Check sheet for the modelled part. Datum: model origin and axes. Units: mm. Face numbers are marked on the shaded views. Round coordinates to 2 decimals unless told otherwise and drop trailing zeros. Order: outer loops, then holes, each group sorted by start corner. A loop starts at its lowest first (then second) coordinate and runs counter-clockwise, first axis right, second up. Notation, with made-up numbers: (87, 51) -> (99, 51) arc R11 ccw to (99, 61) -> close; hole circle Ø3 at (28, 18.5). An arc over 180 degrees is marked (long way). Answer in a Markdown table with one row per item.
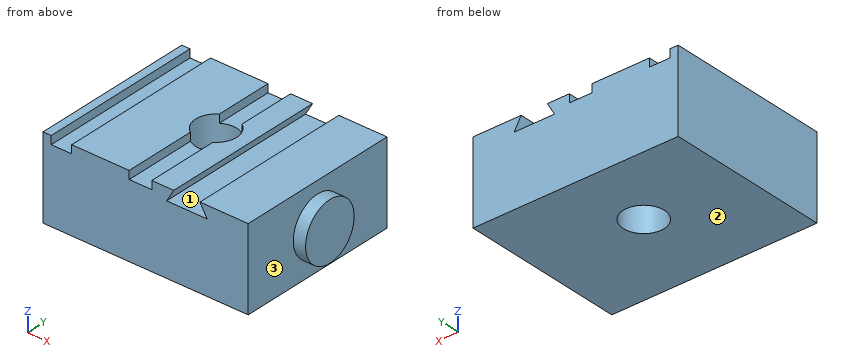
```python
from build123d import *

# Parameters (mm, degrees)
F0_W     = 50
F0_H     = 40
F0_R     = 5
F1_DEPTH = 20
F2_W     = 5
F2_H     = 40
F3_DEPTH = 2
F5_DEPTH = 40.001
F6_R     = 7
F7_DEPTH = 3


with BuildPart() as f1:
    # F0 (on Top) → F1 (new body)
    with BuildSketch(Plane.XY):
        with Locations((1.241206, -1.809668)):
            Rectangle(F0_W, F0_H)
        Circle(F0_R, mode=Mode.SUBTRACT)
    extrude(amount=F1_DEPTH)

    # F2 (on face) → F3 (cut)
    with BuildSketch(Plane.XY.offset(20)):
        with Locations((-19.258794, -1.809668)):
            Rectangle(F2_W, F2_H)
        with BuildLine():
            Line((-2.75, -4.175823), (-2.75, -21.809668))
            Line((-2.75, -21.809668), (2.75, -21.809668))
            Line((2.75, -21.809668), (2.75, -4.175823))
            ThreePointArc((2.75, -4.175823), (0, -5), (-2.75, -4.175823))
        make_face()
        with BuildLine():
            Line((2.75, 18.190332), (-2.75, 18.190332))
            Line((-2.75, 18.190332), (-2.75, 4.175823))
            ThreePointArc((-2.75, 4.175823), (0, 5), (2.75, 4.175823))
            Line((2.75, 4.175823), (2.75, 18.190332))
        make_face()
    extrude(amount=-F3_DEPTH, mode=Mode.SUBTRACT)

    # F4 (on face) → F5 (cut, through all)
    with BuildSketch(Plane.XZ.offset(21.809668)):
        Polygon((14.495603, 20), (8.107771, 20), (6.37572, 17), (16.227654, 17), align=None)
    extrude(amount=-F5_DEPTH, mode=Mode.SUBTRACT)

    # F6 (on face) → F7 (join)
    with BuildSketch(Plane.YZ.offset(26.241206)):
        with Locations((-1.809668, 10)):
            Circle(F6_R)
    extrude(amount=F7_DEPTH)


solid = f1.part
```
(1) Section check D-D on y = -19. Record the boundary of the cut face in (x, z).
Solutions:
| item | result |
|---|---|
| outline | (-23.76, 0) -> (26.24, 0) -> (26.24, 20) -> (14.5, 20) -> (16.23, 17) -> (6.38, 17) -> (8.11, 20) -> (2.75, 20) -> (2.75, 18) -> (-2.75, 18) -> (-2.75, 20) -> (-16.76, 20) -> (-16.76, 18) -> (-21.76, 18) -> (-21.76, 20) -> (-23.76, 20) -> close |
(2) Section check C-C on x = 0. Record the boundary of the cut face in (y, z), plus the area to 3 significant figures.
Solutions:
| item | result |
|---|---|
| outline | (-21.81, 0) -> (-5, 0) -> (-5, 18) -> (-21.81, 18) -> close; (5, 0) -> (18.19, 0) -> (18.19, 18) -> (5, 18) -> close |
| area | 540 mm^2 |
(3) Scan lines: probe 1 along Y at (x, z) = (0, 5.5); probe 2 along X at (y, z) = (0, 13); probe 3 along Z at (x, y) = (13.5, -7). Record each from-to range of solid material in increasing order. Write a range as from..to.
Solutions:
| item | result |
|---|---|
| probe 1 | -21.81..-5, 5..18.19 |
| probe 2 | -23.76..-5, 5..29.24 |
| probe 3 | 0..17 |
(4) Depth check by flat-ended pin: pin 1 Ø0.6 at (y, z) = (13.5, 19) entering from +X; pin 2 Ø1.5 at (x, y) = (-20, -8) entering from +Z; pin 3 Ø8 at (x, y) = (0, 0) entering from -Z. Enter the tip coordinate at first touch or a pass-through.
Solutions:
| item | result |
|---|---|
| pin 1 | x = 26.24 |
| pin 2 | z = 18 |
| pin 3 | through |
(5) Section check A-A on z = 10. Record the boundary of the cut face in (x, y).
Solutions:
| item | result |
|---|---|
| outline | (-23.76, -21.81) -> (26.24, -21.81) -> (26.24, -8.81) -> (29.24, -8.81) -> (29.24, 5.19) -> (26.24, 5.19) -> (26.24, 18.19) -> (-23.76, 18.19) -> close; hole circle Ø10 at (0, 0) |
(6) Section check B-B on y = 3. Record the boundary of the cut face in (x, z), plus the area to 3 significant figures.
Solutions:
| item | result |
|---|---|
| outline | (-23.76, 0) -> (-4, 0) -> (-4, 20) -> (-16.76, 20) -> (-16.76, 18) -> (-21.76, 18) -> (-21.76, 20) -> (-23.76, 20) -> close; (4, 0) -> (26.24, 0) -> (26.24, 4.91) -> (29.24, 4.91) -> (29.24, 15.09) -> (26.24, 15.09) -> (26.24, 20) -> (14.5, 20) -> (16.23, 17) -> (6.38, 17) -> (8.11, 20) -> (4, 20) -> close |
| area | 836 mm^2 |
(7) Draft check along X on the marked faces 1, 2 and 3. Enter one of: pulls with the +X half, pulls with the -X half, needs draft (parallel to the pull), parting line crosses it, or undercut.
Solutions:
| item | result |
|---|---|
| face 1 | undercut |
| face 2 | needs draft |
| face 3 | pulls with the +X half |
